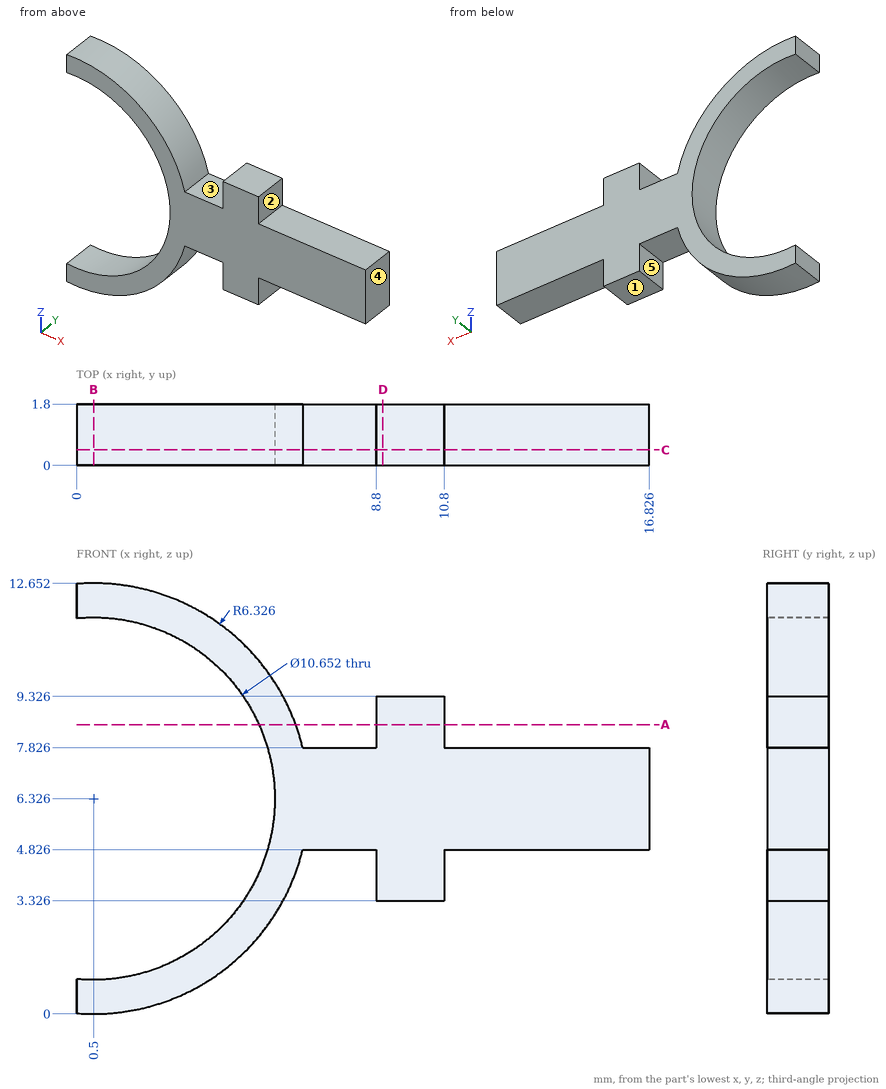
Print and shaded views of the part. All mm, measured from the part's lowest x, y and z. A direction names the side the tool comes from. Coordinates: 2 decimals unless noted, no trailing zeros. Order: outer loops, then holes, each group sorted by start corner. A loop starts at its lowest first (then second) coordinate and runs counter-clockwise, first axis right, second up. Notation, with made-up numbers: (62, -25) - (102, -25) arc R20 cw to (102, -14) - close; hole circle Ø1 at (-28, -21). An arc over 180 degrees is marked (long way). Return JSON: item names as keys, results as strings. Group by question number.
Item 1: Cut at D-D (x = 9). List the corners of the cut face in (y, z), plus the area to 3 significant figures.
Item 2: Cut at A-A (z = 8.5). List the corners of the cut face in (x, y).
Item 3: Cut at C-C (y = 0.45). List the corners of the cut face in (x, z).
Item 4: Cut at B-B (x = 0.5). List the corners of the cut face in (y, z).
Item 5: Drill centre lines: probe 1 along Z at (x, y) = (0.5, 0.85); probe 2 along Z at (x, y) = (13, 1.5); probe 3 along X at (y, z) = (1.3, 8.5). Where is each one in solid material? Low to high. Write a range as from..to.
Item 6: Pin check, flat tips, straight feed: pin 1 (0.9 mm diameter, centred on x = 8, y = 1, fed in from -Z); pin 2 (0.9 mm diameter, centred on x = 7.5, y = 0.5, fed in from +Z); pin 3 (0.9 mm diameter, centred on x = 9.5, y = 0.5, fed in from +Z). Stop position of each tip, or through.
Item 7: Which spindle directions (+Z, -Z, +X, -X, +Y, -Y) get a long thin tool onto all of the face, cutting with end or side? Do the marked faces 1, 2, 3, 4 and 5. Say none if no direction does.
Check values:
{
 "1": {"outline": "(0, 3.33) - (1.8, 3.33) - (1.8, 9.33) - (0, 9.33) - close", "area": "10.8 mm2"},
 "2": {"outline": "(5.36, 0) - (6.44, 0) - (6.44, 1.8) - (5.36, 1.8) - close; (8.8, 0) - (10.8, 0) - (10.8, 1.8) - (8.8, 1.8) - close"},
 "3": {"outline": "(0, 0.02) arc R6.33 ccw to (6.65, 4.83) - (8.8, 4.83) - (8.8, 3.33) - (10.8, 3.33) - (10.8, 4.83) - (16.83, 4.83) - (16.83, 7.83) - (10.8, 7.83) - (10.8, 9.33) - (8.8, 9.33) - (8.8, 7.83) - (6.65, 7.83) arc R6.33 ccw to (0, 12.63) - (0, 11.63) arc R5.33 cw (long way) to (0, 1.02) - close"},
 "4": {"outline": "(0, 0) - (1.8, 0) - (1.8, 1) - (0, 1) - close; (0, 11.65) - (1.8, 11.65) - (1.8, 12.65) - (0, 12.65) - close"},
 "5": {"probe 1": "z = 0..1, 11.65..12.65", "probe 2": "z = 4.83..7.83", "probe 3": "x = 5.36..6.44, 8.8..10.8"},
 "6": {"pin 1": "stops at z = 4.83", "pin 2": "stops at z = 7.83", "pin 3": "stops at z = 9.33"},
 "7": {"face 1": "-Z, +X, +Y, -Y", "face 2": "+Z, +X, +Y, -Y", "face 3": "+Z, +Y, -Y", "face 4": "+Z, -Z, +X, +Y, -Y", "face 5": "-Z, +Y, -Y"}
}
